The drawing under review shows one solid part. Ordinate dimensions are in mm from its lowest x, y, z. A direction names the side the tool comes from. Coordinates: 2 decimals unless noted, no trailing zeros. Order: outer loops, then holes, each group sorted by start corner. A loop starts at its lowest first (then second) coordinate and runs counter-clockwise, first axis right, second up. Notation, with made-up numbers: (15, 58) -> (63, 58) arc R17 cw to (63, 73) -> close; hole circle Ø5 at (46, -8.75). An arc over 180 degrees is marked (long way). Use one line per item in the form item = value.
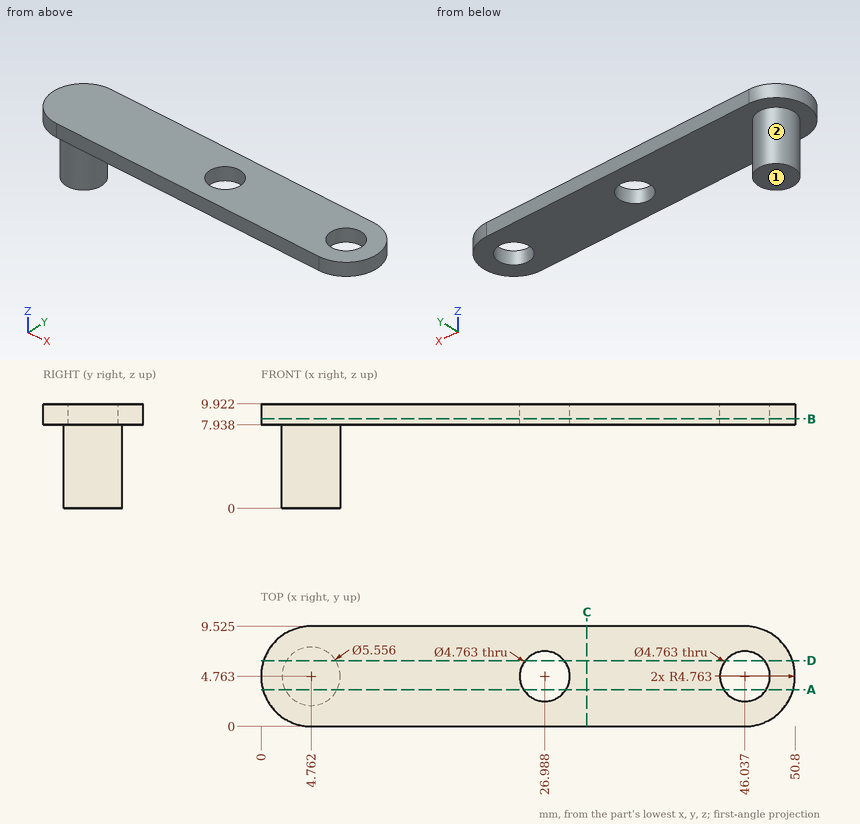
Item 1: Tool access review of the marked faces 1 and 2: name each direction out of +Z, -Z, +X, -X, +Y, -Y from which nothing blocks a thin tool from reaching the whole face with its end or side.
Results found:
face_1 = -Z, +X, -X, +Y, -Y
face_2 = -Z
Item 2: We need section B-B (z = 8.5). Write out the cut boundary in (x, y) (1 decimal), plus the area to 3 significant figures.
Results found:
outline = (4.8, 0) -> (46, 0) arc R4.8 ccw to (46, 9.5) -> (4.8, 9.5) arc R4.8 ccw to start; hole circle Ø4.8 at (27, 4.8); hole circle Ø4.8 at (46, 4.8)
area = 429 mm²
Item 3: We need section C-C (x = 31). Write out the cut boundary in (y, z) (1 decimal), plus the area to 3 significant figures.
Results found:
outline = (0, 7.9) -> (9.5, 7.9) -> (9.5, 9.9) -> (0, 9.9) -> close
area = 18.9 mm²
Item 4: To check wall thickness, follow L1, parallel to X at y = 3.75, z = 8; L2, parallel to Z at x = 23, y = 9; L3, parallel to X at y = 1.25, z = 8.25 (1 decimal). State the ranges of each line that lie inside material, in increasing order. Write a range as from..to.
Results found:
L1 = 0.11..24.83, 29.14..43.88, 48.19..50.69
L2 = 7.94..9.92
L3 = 1.5..49.3
Item 5: Clearance check with flat-ended pins moving along their axes: pin 1 (5.5 mm diameter, centred on x = 26.99, y = 4.76, fed in from -Z); pin 2 (2 mm diameter, centred on y = 7, z = 6.5, fed in from +X); pin 3 (2 mm diameter, centred on x = 10, z = 2, fed in from +Y); pin 4 (2 mm diameter, centred on y = 5.5, z = 4.5, fed in from -X). State where each tip first meets the part, or that it passes through.
Results found:
pin_1 = 7.94
pin_2 = 7.25
pin_3 = through
pin_4 = 1.98
Item 6: We need section A-A (y = 3.5). Write out the cut boundary in (x, z).
Results found:
outline = (0.17, 7.94) -> (2.29, 7.94) -> (2.29, 0) -> (7.24, 0) -> (7.24, 7.94) -> (24.97, 7.94) -> (24.97, 9.92) -> (0.17, 9.92) -> close; (29.01, 7.94) -> (44.02, 7.94) -> (44.02, 9.92) -> (29.01, 9.92) -> close; (48.06, 7.94) -> (50.63, 7.94) -> (50.63, 9.92) -> (48.06, 9.92) -> close
Item 7: We need section D-D (y = 6.25). Write out the cut boundary in (x, z), plus the area to 3 significant figures.
Results found:
outline = (0.24, 7.94) -> (2.42, 7.94) -> (2.42, 0) -> (7.11, 0) -> (7.11, 7.94) -> (25.13, 7.94) -> (25.13, 9.92) -> (0.24, 9.92) -> close; (28.85, 7.94) -> (44.18, 7.94) -> (44.18, 9.92) -> (28.85, 9.92) -> close; (47.9, 7.94) -> (50.56, 7.94) -> (50.56, 9.92) -> (47.9, 9.92) -> close
area = 122 mm²
